Check sheet for the modelled part. Datum: model origin and axes. Units: mm. A direction names the side the tool comes from. Round coordinates to 2 decimals unless told otherwise and drop trailing zeros. Write each loop counter-clockwise with the first axis right and the second up, starting at its lowest first coordinate (ties: lowest second). Pieces come first, ordered by that corner, then holes.
Item 1: Material ranges on line 1 (Y direction, x = -63.5, z = 1.3); line 2 (X direction, y = 14, z = 2.8); line 3 (Y direction, x = -12.7, z = 0.9), recorded low to high.
Item 2: Tool access check on faces 5 (the flat face through (-20, 25.4, 2)), 6 (the cylindrical face through (-75.436, 0.724, 1.61)). Record the directions out of +Z, -Z, +X, -X, +Y, -Y that give a thin tool (end or side, any length) a straight path to the whole face; none if there is none.
Item 3: Release check for a two-part mould opening along Y. For faces 1 (the cylindrical face through (-0.724, 24.636, 1.61)), 2 (the cylindrical face through (-15.058, 11.722, 1.565)), 3 (the cylindrical face through (-60.95, 25.51, 1.57)), 4 (the flat face through (-76.2, 25, 2)) record: +Y half, -Y half, draft (parallel to the pull), parting line (faces both ways), or undercut.
Item 4: Cross-section at C-C on z = 2.25. Enter the section's corners in (x, y), plus the area to 3 significant figures.
Item 5: Cross-section at D-D on x = -63.5. Enter the section's corners in (y, z) (3 decimals).
Item 6: Go/stop test with flat-tipped pins: pin 1 Ø4 at (x, y) = (-38.1, 12.7) entering from -Z; pin 2 Ø1 at (x, z) = (-24.5, 1.5) entering from +Y; pin 3 Ø4 at (x, y) = (-61.5, 8) entering from -Z. Record where each tip stops, or that it passes through.
Item 7: Cross-section at B-B on y = 12.7. Enter the section's corners in (x, z) (3 decimals).
Item 8: Cross-section at A-A on x = -12.7. Enter the section's corners in (y, z) (3 decimals), plus the area to 3 significant figures.
from build123d import *

# Parameters (mm, degrees)
BOSS_EXTRUDE1_DEPTH    = 3.175
F_10_CLEARANCE_HOLE1_D = 5.1054
FILLET1_R              = 2.54


with BuildPart() as part:
    # Sketch1 → Boss-Extrude1 (new body)
    with BuildSketch(Plane.XY):
        Polygon((0, 0), (-76.2, 0), (-76.2, 50.8), (-50.8, 50.8), (-50.8, 38.870384182), (-37.329615818, 25.4), (0, 25.4), align=None)
    extrude(amount=BOSS_EXTRUDE1_DEPTH)

    # #10 Clearance Hole1 (through all)
    with Locations(Plane.XY.offset(3.175)):
        with Locations((-63.5, 38.1), (-63.5, 25.4), (-63.5, 12.7), (-38.1, 12.7), (-25.4, 12.7), (-12.7, 12.7)):
            Hole(F_10_CLEARANCE_HOLE1_D / 2)

    # Fillet1
    fillet1_edges = [part.edges().sort_by_distance(p)[0] for p in [
        (-37.329615818, 25.4, 1.5875),
        (0, 25.4, 1.5875),
        (0, 0, 1.5875),
        (-76.2, 0, 1.5875),
        (-76.2, 50.8, 1.5875),
        (-50.8, 50.8, 1.5875),
        (-50.8, 38.870384182, 1.5875),
    ]]
    fillet(fillet1_edges, radius=FILLET1_R)


solid = part.part
Response values:
1. line 1: y = 0 to 10.15, 15.25 to 22.85, 27.95 to 35.55, 40.65 to 50.8
1. line 2: x = -76.2 to -65.7, -61.3 to -40.3, -35.9 to -27.6, -23.2 to -14.9, -10.5 to 0
1. line 3: y = 0 to 10.15, 15.25 to 25.4
2. face 5: +Z, -Z, +X, +Y
2. face 6: +Z, -Z, -X, -Y
3. face 1: +Y half
3. face 2: undercut
3. face 3: undercut
3. face 4: draft
4. outline: (-76.2, 2.54) arc R2.54 ccw to (-73.66, 0) - (-2.54, 0) arc R2.54 ccw to (0, 2.54) - (0, 22.86) arc R2.54 ccw to (-2.54, 25.4) - (-36.28, 25.4) arc R2.54 cw to (-38.07, 26.14) - (-50.06, 38.13) arc R2.54 cw to (-50.8, 39.92) - (-50.8, 48.26) arc R2.54 ccw to (-53.34, 50.8) - (-73.66, 50.8) arc R2.54 ccw to (-76.2, 48.26) - close; hole circle Ø5.11 at (-63.5, 12.7); hole circle Ø5.11 at (-63.5, 25.4); hole circle Ø5.11 at (-63.5, 38.1); hole circle Ø5.11 at (-38.1, 12.7); hole circle Ø5.11 at (-25.4, 12.7); hole circle Ø5.11 at (-12.7, 12.7)
4. area: 2,540 mm2
5. outline: (0, 0) - (10.147, 0) - (10.147, 3.175) - (0, 3.175) - close; (15.253, 0) - (22.847, 0) - (22.847, 3.175) - (15.253, 3.175) - close; (27.953, 0) - (35.547, 0) - (35.547, 3.175) - (27.953, 3.175) - close; (40.653, 0) - (50.8, 0) - (50.8, 3.175) - (40.653, 3.175) - close
6. pin 1: passes through
6. pin 2: stops at y = 25.4
6. pin 3: stops at z = 0
7. outline: (-76.2, 0) - (-66.053, 0) - (-66.053, 3.175) - (-76.2, 3.175) - close; (-60.947, 0) - (-40.653, 0) - (-40.653, 3.175) - (-60.947, 3.175) - close; (-35.547, 0) - (-27.953, 0) - (-27.953, 3.175) - (-35.547, 3.175) - close; (-22.847, 0) - (-15.253, 0) - (-15.253, 3.175) - (-22.847, 3.175) - close; (-10.147, 0) - (0, 0) - (0, 3.175) - (-10.147, 3.175) - close
8. outline: (0, 0) - (10.147, 0) - (10.147, 3.175) - (0, 3.175) - close; (15.253, 0) - (25.4, 0) - (25.4, 3.175) - (15.253, 3.175) - close
8. area: 64.4 mm2
